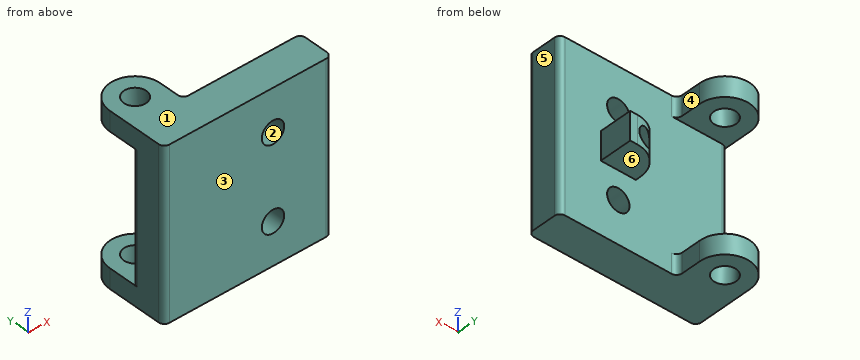
```python
from build123d import *

# Parameters (mm, degrees)
SKETCH1_R               = 4
BOSS_EXTRUDE2_DEPTH     = 7
BOSS_EXTRUDE3_DEPTH     = 23
CUT_EXTRUDE1_DEPTH      = 74.976770002
CUT_EXTRUDE1_DEPTH_BACK = 74.976770002
SKETCH5_R               = 4
SKETCH6_W               = 12.5
SKETCH6_H               = 10
BOSS_EXTRUDE4_DEPTH     = 12.5
FILLET1_R               = 10
SKETCH8_R               = 3
CUT_EXTRUDE2_DEPTH      = 15


with BuildPart() as part:
    # Sketch1 → Boss-Extrude2 (new body)
    with BuildSketch(Plane.XY):
        with BuildLine():
            Line((-37, -11.75), (19, -11.75))
            ThreePointArc((19, -11.75), (20.414213562, -11.164213562), (21, -9.75))
            Line((21, -9.75), (21, -1.25))
            ThreePointArc((21, -1.25), (20.414213562, 0.164213562), (19, 0.75))
            Line((19, 0.75), (-19, 0.75))
            ThreePointArc((-19, 0.75), (-20.414213562, 1.335786438), (-21, 2.75))
            Line((-21, 2.75), (-21, 9.75))
            ThreePointArc((-21, 9.75), (-30, 18.75), (-39, 9.75))
            Line((-39, 9.75), (-39, -9.75))
            ThreePointArc((-39, -9.75), (-38.414213562, -11.164213562), (-37, -11.75))
        make_face()
        with Locations((-30, 9.75)):
            Circle(SKETCH1_R, mode=Mode.SUBTRACT)
    boss_extrude2 = extrude(amount=-BOSS_EXTRUDE2_DEPTH)

    # Sketch4 → Boss-Extrude3 (add)
    with BuildSketch(Plane(origin=(0, 0, -7), x_dir=(-1, 0, 0), z_dir=(0, 0, -1))):
        with BuildLine():
            Line((19, 0.75), (37, 0.75))
            ThreePointArc((37, 0.75), (38.414213562, 0.164213562), (39, -1.25))
            Line((39, -1.25), (39, -9.75))
            ThreePointArc((39, -9.75), (38.414213562, -11.164213562), (37, -11.75))
            Line((37, -11.75), (-19, -11.75))
            ThreePointArc((-19, -11.75), (-20.414213562, -11.164213562), (-21, -9.75))
            Line((-21, -9.75), (-21, -1.25))
            ThreePointArc((-21, -1.25), (-20.414213562, 0.164213562), (-19, 0.75))
            Line((-19, 0.75), (19, 0.75))
        make_face()
    boss_extrude3 = extrude(amount=BOSS_EXTRUDE3_DEPTH)

    # Mirror2: Boss-Extrude3 across plane
    add(boss_extrude3.mirror(Plane(origin=(0, 0, -30), x_dir=(1, 0, 0), z_dir=(0, 0, -1))))

    # Mirror3: Boss-Extrude2 across plane
    add(boss_extrude2.mirror(Plane(origin=(0, 0, -30), x_dir=(1, 0, 0), z_dir=(0, 0, -1))))

    # Sketch5 → Cut-Extrude1 (cut, two sides: drawn at the far end of the back side and taken through both)
    with BuildSketch(Plane(origin=(0, 0, 0), x_dir=(1, 0, 0), z_dir=(0, 1, 0)).offset(-CUT_EXTRUDE1_DEPTH_BACK)):
        with Locations(Location((0, 45, 0), (0, 0, 270))):
            Circle(SKETCH5_R)
        with Locations(Location((0, 15, 0), (0, 0, 270))):
            Circle(SKETCH5_R)
    extrude(amount=CUT_EXTRUDE1_DEPTH + CUT_EXTRUDE1_DEPTH_BACK, mode=Mode.SUBTRACT)

    # Sketch6 → Boss-Extrude4 (add)
    with BuildSketch(Plane(origin=(0, 0, 0), x_dir=(1, 0, 0), z_dir=(0, 1, 0))):
        with Locations((0, 30)):
            Rectangle(SKETCH6_W, SKETCH6_H)
    extrude(amount=BOSS_EXTRUDE4_DEPTH)

    # Fillet1
    fillet1_edges = [part.edges().sort_by_distance(p)[0] for p in [
        (-6.25, 12.5, -30),
    ]]
    fillet(fillet1_edges, radius=FILLET1_R)

    # Sketch8 → Cut-Extrude2 (cut)
    with BuildSketch(Plane(origin=(0, 12.5, 0), x_dir=(1, 0, 0), z_dir=(0, 1, 0))):
        with Locations(Location((0, 30, 0), (0, 0, 270))):
            Circle(SKETCH8_R)
    extrude(amount=-CUT_EXTRUDE2_DEPTH, mode=Mode.SUBTRACT)


solid = part.part
```
Work out the finished part from the listing and answer in its coordinate system (mm). Face numbers are marked on the shaded views. A direction names the side the tool comes from. Round coordinates to 2 decimals unless told otherwise and drop trailing zeros. Loops run counter-clockwise (first coordinate to the right, second up) from the corner with the lowest first, then second, coordinate; pieces in that order, holes last. Notation, with made-up numbers: (-6, 63.5) -> (28, 63.5) arc R12 ccw to (28, 73.5) -> close; hole circle Ø3 at (-4.5, 68). An arc over 180 degrees is marked (long way). Write each question's results on one line, items separated by ' | '. Start each with the question number.
1. Given pin 1 Ø5 at (x, z) = (0, -30) entering from +Y; pin 2 Ø0.9 at (y, z) = (1.5, -30) entering from -X; pin 3 Ø12 at (x, z) = (-10, -15.5) entering from +Y, each flat-ended and moving along its own axis, determine where each tip first touches the part or whether it passes through.
2. For a pull along Z with two mould halves and no side action, classify the marked faces 1, 2 and 3 as +Z half, -Z half, draft (parallel to the pull), parting line (faces both ways), or undercut.
3. Section A-A (z = -45) is taken. Determine the outline of the cut face in (x, y).
4. Section B-B (x = -30) is taken. Determine the outline of the cut face in (y, z), plus the area to 3 significant figures.
5. A tool of negligible diameter and unlimited length cuts with its end or side. For the marked faces 4, 5 and 6, from which of +Z, -Z, +X, -X, +Y, -Y can it reach the whole face along a straight path? Write none if from no direction.
6. Section C-C (y = 17) is taken. Determine the outline of the cut face in (x, z), plus the area to 3 significant figures.
7. Find the intervals of material crossed by probe 1 along Y at (x, z) = (-30, -57); probe 2 along Z at (x, y) = (-28, 17); probe 3 along X at (y, z) = (-8.75, -15), in increasing order. Write a range as from..to.
8. Section D-D (y = 4) is taken. Determine the outline of the cut face in (x, z), plus the area to 3 significant figures.
Evaluation:
1) pin 1: stops at y = -2.5 | pin 2: stops at x = -6.25 | pin 3: stops at y = 0.75
2) face 1: +Z half | face 2: undercut | face 3: draft
3) outline: (-39, -9.75) arc R2 ccw to (-37, -11.75) -> (-4, -11.75) -> (-4, 0.75) -> (-37, 0.75) arc R2 ccw to (-39, -1.25) -> close; (4, -11.75) -> (19, -11.75) arc R2 ccw to (21, -9.75) -> (21, -1.25) arc R2 ccw to (19, 0.75) -> (4, 0.75) -> close
4) outline: (-11.75, -60) -> (5.75, -60) -> (5.75, -53) -> (0.75, -53) -> (0.75, -7) -> (5.75, -7) -> (5.75, 0) -> (-11.75, 0) -> close; (13.75, -60) -> (18.75, -60) -> (18.75, -53) -> (13.75, -53) -> close; (13.75, -7) -> (18.75, -7) -> (18.75, 0) -> (13.75, 0) -> close | area: 890 mm2
5) face 4: +Z, -Z, +X, +Y | face 5: +Z, -Z, +X, +Y, -Y | face 6: -Z, +X, -X, +Y
6) outline: (-35.33, -60) -> (-24.67, -60) -> (-24.67, -53) -> (-35.33, -53) -> close; (-35.33, -7) -> (-24.67, -7) -> (-24.67, 0) -> (-35.33, 0) -> close | area: 149 mm2
7) probe 1: y = -11.75..5.75, 13.75..18.75 | probe 2: z = -60..-53, -7..0 | probe 3: x = -39..-4, 4..21
8) outline: (-39, -60) -> (-21, -60) -> (-21, -53) -> (-39, -53) -> close; (-39, -7) -> (-21, -7) -> (-21, 0) -> (-39, 0) -> close; (-6.14, -35) -> (6.25, -35) -> (6.25, -25) -> (-6.14, -25) -> close; hole circle Ø6 at (0, -30) | area: 348 mm2
